Here's how the part is built. I have some questions about the finished solid (model axes, mm). A direction names the side the tool comes from. Give positions to 0.01 mm unless a question says otherwise; leave off trailing zeros. Write each loop counter-clockwise with the first axis right and the second up, starting at its lowest first coordinate (ties: lowest second). Pieces come first, ordered by that corner, then holes. Notation, with made-up numbers: (28.25, 61) - (36.25, 61) arc R19 ccw to (36.25, 81) - close; hole circle Ø2 at (43.5, -30.5). An arc over 180 degrees is marked (long way). Use a Markdown table: item, result.
```python
from build123d import *

# Parameters (mm, degrees)
CUT_EXTRUDE1_DEPTH      = 14.868123463
CUT_EXTRUDE1_DEPTH_BACK = 14.868123463
SKETCH2_R               = 1.5
SCALE1_SCALE            = 1.5


with BuildPart() as part:
    # Sketch1 → Revolve1 (revolve)
    with BuildSketch(Plane.XY, mode=Mode.PRIVATE) as revolve1_sk:
        Polygon((0, 9.712098042), (-6.25, 9.712098042), (-6.25, 8.712098042), (-7, 8.712098042), (-7, -5.287901958), (-6.25, -5.287901958), (-4.75, -1.166685828), (-4.75, 5.712098042), (0, 8.566185983), align=None)
    revolve(revolve1_sk.sketch.rotate(Axis((0, 2.420801252, 0), (0, 1, 0)), 270), axis=Axis((0, 2.420801252, 0), (0, 1, 0)))

    # Sketch2 → Cut-Extrude1 (cut, two sides: drawn at the far end of the back side and taken through both)
    with BuildSketch(Plane.XY.offset(-CUT_EXTRUDE1_DEPTH_BACK)):
        with Locations((0, 1.712098042)):
            Circle(SKETCH2_R)
    extrude(amount=CUT_EXTRUDE1_DEPTH + CUT_EXTRUDE1_DEPTH_BACK, mode=Mode.SUBTRACT)


with BuildPart() as part_1:
    # Scale1: scaled about (3.5175e-05, 3.523748347, -7.815e-06)
    add(part.part.scale(SCALE1_SCALE).moved(Location((-1.7588e-05, -1.761874174, 3.908e-06))))


solid = part_1.part
```
Item 1: If we section it at A-A, the plane y = 2.25: Write out the boundary of the cut face in (x, z) (3 decimals).
Values:
| item | result |
|---|---|
| outline | (-1.726, -10.357) - (-1.726, -6.913) arc R7.125 cw to (-1.726, 6.913) - (-1.726, 10.357) arc R10.5 ccw to start; (1.726, -10.357) arc R10.5 ccw to (1.726, 10.357) - (1.726, 6.913) arc R7.125 cw to (1.726, -6.913) - close |
Item 2: Thinking about a two-plate mould opening in Z: for faces 4 (the conical face through (-0.3, 10.4, -1.1)), 5 (the cylindrical face through (5.705, 12.046, 7.44)), 6 (the cylindrical face through (2.146, 1.482, 8.607)), which applies, +Z half, -Z half, draft (parallel to the pull), parting line (faces both ways), or undercut?
Values:
| item | result |
|---|---|
| face 4 | undercut |
| face 5 | parting line |
| face 6 | draft |
Item 3: If we section it at B-B, the plane y = -6: Write out the boundary of the cut face in (x, z).
Values:
| item | result |
|---|---|
| outline | circle Ø21 at (0, 0); hole circle Ø16.06 at (0, 0) |
Item 4: Will these pins go through, and if not, where does the flat tip stop? pin 1 Ø4 at (x, y) = (5, 7) entering from +Z; pin 2 Ø8 at (x, y) = (6.5, 2.5) entering from +Z; pin 3 Ø1 at (x, y) = (7, -7.5) entering from +Z.
Values:
| item | result |
|---|---|
| pin 1 | stops at z = 10.06 |
| pin 2 | stops at z = 10.2 |
| pin 3 | stops at z = 8.25 |
Item 5: For faces 1 (the flat face through (0, 12.806, 0)), 2 (the cylindrical face through (2.73, 1.72, -6.58)), 3 (the flat face through (-9, 11.306, -4)), which set-ups out of +Z, -Z, +X, -X, +Y, -Y let a thin tool reach every point of the face, with its end or its side?
Values:
| item | result |
|---|---|
| face 1 | +Z, -Z, +X, -X, +Y |
| face 2 | -Y |
| face 3 | +Y |
Item 6: If we section it at C-C, the plane y = 8: Write out the boundary of the cut face in (x, z), plus the area to 3 significant figures.
Values:
| item | result |
|---|---|
| outline | circle Ø21 at (0, 0); hole circle Ø10.28 at (0, 0) |
| area | 263 mm2 |
Item 7: I need wall thicknesses on line 1 along Y through (x, z) = (9, 4.75); line 2 along Z through (x, y) = (2, 3.5); line 3 along X through (y, z) = (-4.5, -2.25). Which ranges of each line are inside material? Lowest first, please. Write a range as [from, to].
Values:
| item | result |
|---|---|
| line 1 | y = [-9.69, 11.31] |
| line 2 | z = [-10.31, -6.84], [6.84, 10.31] |
| line 3 | x = [-10.26, -7.14], [7.14, 10.26] |
